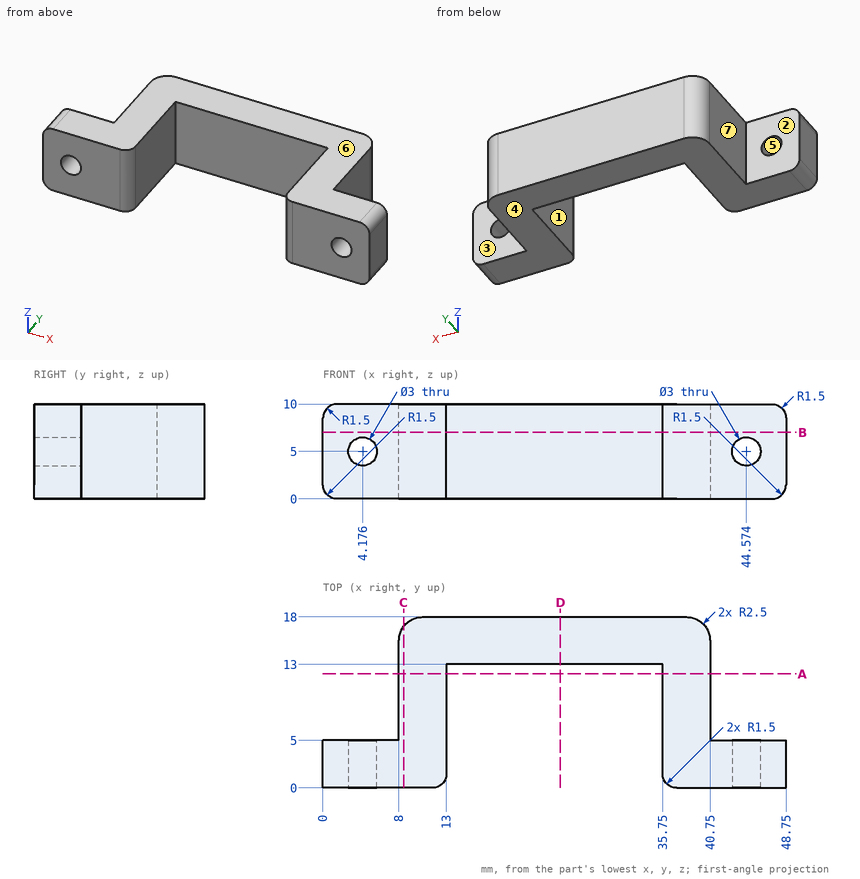
Print and shaded views of the part. All mm, measured from the part's lowest x, y and z. A direction names the side the tool comes from. Give positions to 0.01 mm unless a question says otherwise; leave off trailing zeros. Write each loop counter-clockwise with the first axis right and the second up, starting at its lowest first coordinate (ties: lowest second). Pieces come first, ordered by that corner, then holes. Notation, with made-up numbers: (57.25, -29.75) -> (100.25, -29.75) arc R15 cw to (100.25, -15.75) -> close; hole circle Ø5 at (-22, 28.25). An arc over 180 degrees is marked (long way). Use CSV: the item, a comma, the result in double quotes. Start each with the question number.
1) Tool access for the marked faces 1, 2 and 3: list every direction of +Z, -Z, +X, -X, +Y, -Y with a clear straight run to the whole face (end or side of a thin tool).
2) Cut at B-B on z = 7. List the corners of the cut face in (x, y), plus the area to 3 significant figures.
3) Two-plate mould, pull along Z, no slides. Class the marked faces 4, 5, 6 and 7: released by +Z, released by -Z, zero draft, split by the parting line, or undercut.
4) Drill centre lines: L1, parallel to X at y = 7, z = 5.75; L2, parallel to Y at x = 43.5, z = 8.75; L3, parallel to Y at x = 30, z = 2.25. Where is each one in solid material? Low to high.
5) Cut at A-A on y = 12. List the corners of the cut face in (x, z), plus the area to 3 significant figures.
6) Cut at C-C on x = 8.5. List the corners of the cut face in (y, z), plus the area to 3 significant figures.
7) Pin check, flat tips, straight feed: P1, Ø2.5, axis at x = 44.5, z = 4, coming from the +Y side; P2, Ø1, axis at y = 7, z = 6, coming from the -X side; P3, Ø3, axis at x = 33.5, z = 1.5, coming from the -Y side; P4, Ø1.8, axis at x = 4.18, z = 5, coming from the +Y side. Stop position of each tip, or through.
8) Cut at D-D on x = 25. List the corners of the cut face in (y, z), plus the area to 3 significant figures.
Final values:
1,face 1,"+Z, -Z, -Y"
1,face 2,"+Z, -Z, -X, +Y"
1,face 3,"+Z, -Z, +X, +Y"
2,outline,"(0, 0) -> (11.5, 0) arc R1.5 ccw to (13, 1.5) -> (13, 13) -> (35.75, 13) -> (35.75, 1.5) arc R1.5 ccw to (37.25, 0) -> (48.75, 0) -> (48.75, 5) -> (40.75, 5) -> (40.75, 15.5) arc R2.5 ccw to (38.25, 18) -> (10.5, 18) arc R2.5 ccw to (8, 15.5) -> (8, 5) -> (0, 5) -> close"
2,area,"370 mm2"
3,face 4,"released by -Z"
3,face 5,"undercut"
3,face 6,"released by +Z"
3,face 7,"zero draft"
4,L1,"x = 8 to 13, 35.75 to 40.75"
4,L2,"y = 0 to 5"
4,L3,"y = 13 to 18"
5,outline,"(8, 0) -> (13, 0) -> (13, 10) -> (8, 10) -> close; (35.75, 0) -> (40.75, 0) -> (40.75, 10) -> (35.75, 10) -> close"
5,area,"100 mm2"
6,outline,"(0, 0) -> (17, 0) -> (17, 10) -> (0, 10) -> close"
6,area,"170 mm2"
7,P1,"stops at y = 5"
7,P2,"stops at x = 8"
7,P3,"stops at y = 13"
7,P4,"passes through"
8,outline,"(13, 0) -> (18, 0) -> (18, 10) -> (13, 10) -> close"
8,area,"50.0 mm2"
